Source: CAD feature listing. Evaluate the final solid. Frame: model axes, mm. A direction names the side the tool comes from. Give positions to 0.01 mm unless a question says otherwise; leave off trailing zeros. Order: outer loops, then holes, each group sorted by start corner. A loop starts at its lowest first (then second) coordinate and runs counter-clockwise, first axis right, second up.
1) Section B-B, the plane x = 140.5. Return loops of the section in (y, z), plus the area to 3 significant figures.
2) Draft query along Y for faces 4 (the face through (76, -74.6, -95)), 5 (the face through (73.881, 69.177, 21.512)), 6 (the face through (137.4, -3, -86)). Return one class per face: released by +Y, released by -Y, zero draft, split by the parting line, or undercut.
3) Material intervals for line 1 (Z direction, x = 45.5, y = -15.5); line 2 (Z direction, x = 55, y = 25.5); line 3 (Y direction, x = 31.5, z = 57), sorted ascending.
4) Access query for faces 1 (the face through (75.979, 28.172, -46.252)), 2 (the face through (74, 9, -93.485)), 3 (the face through (76, 78, -102)). Directions: +Z, -Z, +X, -X, +Y, -Y. A direction counts if a zero-diameter tool reaches every point of the face in a straight line with its end or side. Return the directions, or none.
5) First-contact query: P1, Ø12, axis at x = 37, z = -69.5, coming from the +Y side; P2, Ø5, axis at x = 120.5, y = 21, coming from the +Z side; P3, Ø3, axis at x = 42, z = -32, coming from the +Y side. Flat tips, straight axial feed; report the tip coordinate or a pass-through.
6) Section D-D, the plane x = 61. Return loops of the section in (y, z).
7) Section A-A, the plane y = 47. Return loops of the section in (x, z).
8) Section C-C, the plane y = 21. Return loops of the section in (x, z).
```python
from build123d import *

# Parameters (mm, degrees)
F1_DEPTH = 149.86
F3_DEPTH = 149.86
F5_DEPTH = 149.86
F7_DEPTH = 149.86
F8_W     = 128.3415369689
F8_H     = 15.6382545829
F9_DEPTH = 124.714


with BuildPart() as f1:
    # F0 (on Right) → F1 (new body)
    with BuildSketch(Plane.YZ):
        with BuildLine():
            Line((44.2407907503, 110.8653195666), (-72.9446343889, -105.8618834673))
            Line((-72.9446343889, -105.8618834673), (39.9045087847, -105.8618834673))
            ThreePointArc((39.9045087847, -105.8618834673), (23.7226648403, -80.0116112868), (12.4027548979, -51.6929198598))
            ThreePointArc((12.4027548979, -51.6929198598), (16.7125207221, -18.6962392489), (44.2407907503, 0))
            ThreePointArc((44.2407907503, 0), (69.4384780949, 21.9062796628), (79.5394011802, 53.7304825436))
            ThreePointArc((79.5394011802, 53.7304825436), (68.2833280218, 86.247719056), (44.2407907503, 110.8653195666))
        make_face()
    extrude(amount=F1_DEPTH)

    # F2 (on face) → F3 (join)
    with BuildSketch(Plane.YZ.offset(149.86)):
        with BuildLine():
            ThreePointArc((-68.2184364909, -97.1210724816), (-74.6761266058, -94.9578371945), (-80.0221942177, -90.738724774))
            Line((-80.0221942177, -90.738724774), (-84.7749029282, -99.5285658693))
            ThreePointArc((-84.7749029282, -99.5285658693), (-79.6540711296, -104.1789354389), (-72.9446343889, -105.8618834673))
            Line((-72.9446343889, -105.8618834673), (-68.2184364909, -97.1210724816))
        make_face()
        with BuildLine():
            ThreePointArc((-50.4522174888, -64.2635481928), (-47.7805051422, -86.9400572359), (-68.2184364909, -97.1210724816))
            Line((-68.2184364909, -97.1210724816), (-72.9446343889, -105.8618834673))
            Line((-72.9446343889, -105.8618834673), (39.9045087847, -105.8618834673))
            ThreePointArc((39.9045087847, -105.8618834673), (23.7226648403, -80.0116112868), (12.4027548979, -51.6929198598))
            ThreePointArc((12.4027548979, -51.6929198598), (16.7125207221, -18.6962392489), (44.2407907503, 0))
            ThreePointArc((44.2407907503, 0), (69.4384780949, 21.9062796628), (79.5394011802, 53.7304825436))
            ThreePointArc((79.5394011802, 53.7304825436), (68.2833280218, 86.247719056), (44.2407907503, 110.8653195666))
            Line((44.2407907503, 110.8653195666), (-50.4522174888, -64.2635481928))
        make_face()
    extrude(amount=-F3_DEPTH)

    # F4 (on face) → F5 (join)
    with BuildSketch(Plane.YZ.offset(149.86)):
        with BuildLine():
            ThreePointArc((12.4027548979, -51.6929198598), (21.3713458152, -75.1942598568), (33.6986931702, -97.1210724816))
            Line((33.6986931702, -97.1210724816), (78.4184666755, -97.1210724816))
            ThreePointArc((78.4184666755, -97.1210724816), (31.1006677255, -59.1983474365), (44.2407907503, 0))
            ThreePointArc((44.2407907503, 0), (16.7125207221, -18.6962392489), (12.4027548979, -51.6929198598))
        make_face()
    extrude(amount=-F5_DEPTH)

    # F6 (on face) → F7 (join)
    with BuildSketch(Plane.YZ.offset(149.86)):
        with BuildLine():
            Line((78.0001431704, -97.1210724816), (33.6986931702, -97.1210724816))
            ThreePointArc((33.6986931702, -97.1210724816), (36.7329195442, -101.5402405334), (39.9045087847, -105.8618834673))
            Line((39.9045087847, -105.8618834673), (78.0001431704, -105.8618834673))
            Line((78.0001431704, -105.8618834673), (78.0001431704, -97.1210724816))
        make_face()
    extrude(amount=-F7_DEPTH)

    # F8 (on face) → F9 (cut)
    with BuildSketch(Plane(origin=(0, 78.0001431704, 0), x_dir=(-1, 0, 0), z_dir=(0, 1, 0))):
        with Locations((-73.2293818146, -85.6656767428)):
            Rectangle(F8_W, F8_H)
    extrude(amount=-F9_DEPTH, mode=Mode.SUBTRACT)


solid = f1.part
```
From the geometry:
1. outline: (-84.77, -99.53) arc R14.22 ccw to (-72.94, -105.86) - (78, -105.86) - (78, -97.12) - (78.42, -97.12) arc R57.37 cw to (44.24, 0) arc R61.72 ccw to (79.54, 53.73) arc R78.78 ccw to (44.24, 110.87) - (-68.22, -97.12) arc R19.85 cw to (-80.02, -90.74) - close
1. area: 15,100 mm2
2. face 4: undercut
2. face 5: released by +Y
2. face 6: zero draft
3. line 1: z = -105.86 to -93.48, -77.85 to 0.38
3. line 2: z = -105.86 to -93.48, -77.85 to 76.21
3. line 3: y = 15.12 to 79.1
4. face 1: +X, -X, +Y
4. face 2: +Y
4. face 3: -Z, +X, -X, +Y
5. P1: stops at y = 40.03
5. P2: stops at z = 72.51
5. P3: stops at y = 28.67
6. outline: (-84.77, -99.53) arc R14.22 ccw to (-72.94, -105.86) - (78, -105.86) - (78, -97.12) - (78.42, -97.12) arc R57.37 cw to (64.07, -93.48) - (-46.71, -93.48) - (-46.71, -77.85) - (41.97, -77.85) arc R57.37 cw to (44.24, 0) arc R61.72 ccw to (79.54, 53.73) arc R78.78 ccw to (44.24, 110.87) - (-68.22, -97.12) arc R19.85 cw to (-80.02, -90.74) - close
7. outline: (0, -105.86) - (149.86, -105.86) - (149.86, -82.94) - (137.4, -82.94) - (137.4, -93.48) - (9.06, -93.48) - (9.06, -82.94) - (0, -82.94) - close; (0, 1.39) - (149.86, 1.39) - (149.86, 108.98) - (0, 108.98) - close
8. outline: (0, -105.86) - (149.86, -105.86) - (149.86, 67.88) - (0, 67.88) - close; hole (9.06, -93.48) - (137.4, -93.48) - (137.4, -77.85) - (9.06, -77.85) - close
